The listing builds one solid part. Answer for the finished solid, in the listing's coordinates (mm). Face numbers are marked on the shaded views. A direction names the side the tool comes from. Coordinates: 2 decimals unless noted, no trailing zeros. Order: outer loops, then holes, each group sorted by start corner. A loop starts at its lowest first (then second) coordinate and runs counter-clockwise, first axis right, second up. Notation, with made-up numbers: (-10, 62.25) -> (32, 62.25) arc R14 ccw to (32, 75.25) -> close; hole circle Ø9 at (-31.5, 59.5). An arc over 180 degrees is marked (long way). Answer in a Markdown table with one row per item. Add a question column.
Autodesk Inventor part; units mm, degrees
ref_plane "Work Plane1" through (0, 6, 0) normal (0, 1, 0) x (1, 0, 0)
ref_plane "YZ Plane" through (0, 0, 0) normal (1, 0, 0) x (0, 1, 0)
ref_plane "XZ Plane" through (0, 0, 0) normal (0, 1, 0) x (-1, 0, 0)
sketch "Sketch1" plane through (0, 0, 0) normal (0, 1, 0) x (-1, 0, 0)
  circle A0 centre (0, 22.5) radius 3.5
  line L0 (0, 30) -> (4, 30)
  line L1 (4, 30) -> (9.4194, 15.3387)
  line L2 (0, 30) -> (-4, 30)
  line L3 (-4, 30) -> (-9.4194, 15.3387)
  circle A1 centre (0, -22.5) radius 3.5
  line L4 (0, -30) -> (4, -30)
  line L5 (4, -30) -> (9.4194, -15.3387)
  line L6 (0, -30) -> (-4, -30)
  line L7 (-4, -30) -> (-9.4194, -15.3387)
  arc A2 (-9.4194, 15.3387) -> (-9.4194, -15.3387) centre (0, 0) ccw
  arc A3 (9.4194, -15.3387) -> (9.4194, 15.3387) centre (0, 0) ccw
extrude "Extrusion1" add sketch "Sketch1" along normal blind 6
ref_plane "Work Plane1" through (0, 6, 0) normal (0, 1, 0) x (1, 0, 0)
sketch "Sketch2" plane through (0, 6, 0) normal (0, 1, 0) x (1, 0, 0)
  circle A0 centre (0, 0) radius 17.5
  circle A1 centre (0, 0) radius 16.5
  dimension "d9" = 35
  dimension "d12" = 33
extrude "Extrusion2" add sketch "Sketch2" along normal blind 5
sketch "Sketch3" plane through (0, 6, 0) normal (0, 1, 0) x (1, 0, 0)
  circle A0 centre (0, 0) radius 5
  circle A1 centre (0, 0) radius 6
  dimension "d15" = 10
  dimension "d16" = 12
extrude "Extrusion3" add sketch "Sketch3" along normal blind 10
properties part number "Chumacera con rodamiento 10 mm kfl000"
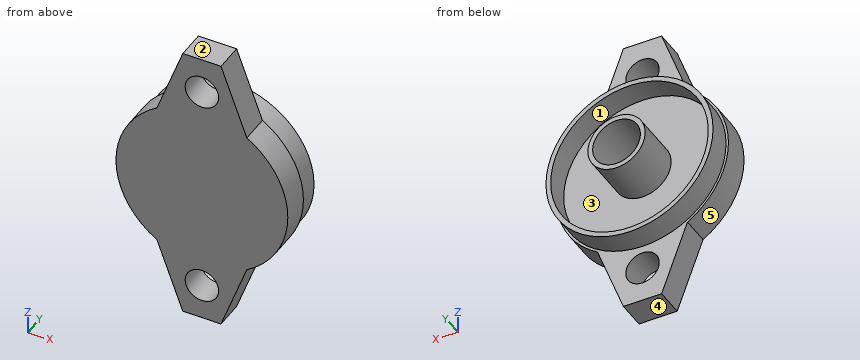
Q1. A cutting plane is placed at C-C (x = 0). Determine the outline of the cut face in (y, z).
Q2. Determine the mould class of the marked faces 3, 4 and 5 for opening direction X: +X half, -X half, draft (parallel to the pull), parting line (faces both ways), or undercut.
Q3. Given pin 1 (1 mm diameter, centred on y = 8, z = -13.5, fed in from +X); pin 2 (1 mm diameter, centred on x = -13.5, z = -8.5, fed in from -Y); pin 3 (4 mm diameter, centred on y = 11.5, z = -7, fed in from -X); pin 4 (8 mm diameter, centred on x = 9.5, y = 11.5, fed in from -Z), each flat-ended and moving along its own axis, determine where each tip first touches the part or whether it passes through.
Q4. A cutting plane is placed at D-D (z = 22.5). Determine the outline of the cut face in (x, y), then the cut area to 3 significant figures.
Q5. A cutting plane is placed at B-B (z = 0). Determine the outline of the cut face in (x, y), then the cut area to 3 significant figures.
Q6. A cutting plane is placed at A-A (y = 6.75). Determine the outline of the cut face in (x, z).
Q7. For the marked faces 1 and 2, determine the directions among +Z, -Z, +X, -X, +Y, -Y from which every point of the face is accessible in a straight line to the end or side of a thin tool.
Q8. Straight lines are drawn through the part: line 1 (Z direction, x = 0, y = 9.15); line 2 (Z direction, x = 0, y = 1.45). For each, find the intervals that lie inside material, in ascending order.
Returned:
| question | item | result |
|---|---|---|
| 1 | outline | (0, -30) -> (6, -30) -> (6, -26) -> (0, -26) -> close; (0, -19) -> (6, -19) -> (6, -17.5) -> (11, -17.5) -> (11, -16.5) -> (6, -16.5) -> (6, -6) -> (16, -6) -> (16, -5) -> (6, -5) -> (6, 5) -> (16, 5) -> (16, 6) -> (6, 6) -> (6, 16.5) -> (11, 16.5) -> (11, 17.5) -> (6, 17.5) -> (6, 19) -> (0, 19) -> close; (0, 26) -> (6, 26) -> (6, 30) -> (0, 30) -> close |
| 2 | face 3 | undercut |
| 2 | face 4 | draft |
| 2 | face 5 | -X half |
| 3 | pin 1 | stops at x = 11.72 |
| 3 | pin 2 | stops at y = 0 |
| 3 | pin 3 | stops at x = -16.75 |
| 3 | pin 4 | stops at z = -16.6 |
| 4 | outline | (-6.77, 0) -> (-3.5, 0) -> (-3.5, 6) -> (-6.77, 6) -> close; (3.5, 0) -> (6.77, 0) -> (6.77, 6) -> (3.5, 6) -> close |
| 4 | area | 39.3 mm² |
| 5 | outline | (-18, 0) -> (18, 0) -> (18, 6) -> (17.5, 6) -> (17.5, 11) -> (16.5, 11) -> (16.5, 6) -> (6, 6) -> (6, 16) -> (5, 16) -> (5, 6) -> (-5, 6) -> (-5, 16) -> (-6, 16) -> (-6, 6) -> (-16.5, 6) -> (-16.5, 11) -> (-17.5, 11) -> (-17.5, 6) -> (-18, 6) -> close |
| 5 | area | 246 mm² |
| 6 | outline | circle Ø35 at (0, 0); circle Ø12 at (0, 0); hole circle Ø33 at (0, 0); hole circle Ø10 at (0, 0) |
| 7 | face 1 | +Y |
| 7 | face 2 | +Z, +X, -X, +Y, -Y |
| 8 | line 1 | z = -17.5 to -16.5, -6 to -5, 5 to 6, 16.5 to 17.5 |
| 8 | line 2 | z = -30 to -26, -19 to 19, 26 to 30 |
